For this review, take the finished solid that the model builds, in its own axes (mm). A direction names the side the tool comes from. Give positions to 0.01 mm unless a question says otherwise; leave off trailing zeros. Write each loop counter-clockwise with the first axis right and the second up, starting at its lowest first coordinate (ties: lowest second). Pieces come first, ordered by that corner, then holes. Notation, with made-up numbers: (17.25, -1) -> (61.25, -1) arc R21 cw to (61.25, 29) -> close; hole circle Ø7 at (33.25, -16). An arc over 180 degrees is marked (long way). Return JSON: item names as keys, results as strings.
from build123d import *

# Parameters (mm, degrees)
SKETCH_3_R          = 13
EXTRUDE_1_DEPTH     = 5
CUT_EXTRUDE_2_DEPTH = 2.5
SKETCH_11_R         = 10
EXTRUDE_2_DEPTH     = 15
SKETCH_6_R          = 2
CUT_EXTRUDE_3_DEPTH = 33
SKETCH_7_R          = 7
CUT_EXTRUDE_4_DEPTH = 23
CUT_EXTRUDE_6_DEPTH = 5
FILLET_1_R          = 1
SKETCH_10_W         = 2
SKETCH_10_H         = 14
CUT_EXTRUDE_7_DEPTH = 0.5


with BuildPart() as part:
    # ｽｹｯﾁ3 → ﾎﾞｽ - 押し出し1 (new body)
    with BuildSketch(Plane.XY):
        Circle(SKETCH_3_R)
    extrude(amount=EXTRUDE_1_DEPTH)

    # ｽｹｯﾁ2 → ｶｯﾄ - 押し出し2 (cut)
    with BuildSketch(Plane.XY):
        with BuildLine():
            Line((3.75, 6.495190528), (2.463350586, 13.926501921))
            ThreePointArc((2.463350586, 13.926501921), (0, 16), (-2.463350586, 13.926501921))
            Line((-2.463350586, 13.926501921), (-3.75, 6.495190528))
            Line((-3.75, 6.495190528), (-10.829029157, 9.096575147))
            ThreePointArc((-10.829029157, 9.096575147), (-13.856406461, 8), (-13.292379743, 4.829926775))
            Line((-13.292379743, 4.829926775), (-7.5, 0))
            Line((-7.5, 0), (-13.292379743, -4.829926775))
            ThreePointArc((-13.292379743, -4.829926775), (-13.856406461, -8), (-10.829029157, -9.096575147))
            Line((-10.829029157, -9.096575147), (-3.75, -6.495190528))
            Line((-3.75, -6.495190528), (-2.463350586, -13.926501921))
            ThreePointArc((-2.463350586, -13.926501921), (0, -16), (2.463350586, -13.926501921))
            Line((2.463350586, -13.926501921), (3.75, -6.495190528))
            Line((3.75, -6.495190528), (10.829029157, -9.096575147))
            ThreePointArc((10.829029157, -9.096575147), (13.856406461, -8), (13.292379743, -4.829926775))
            Line((13.292379743, -4.829926775), (7.5, 0))
            Line((7.5, 0), (13.292379743, 4.829926775))
            ThreePointArc((13.292379743, 4.829926775), (13.856406461, 8), (10.829029157, 9.096575147))
            Line((10.829029157, 9.096575147), (3.75, 6.495190528))
        make_face()
    extrude(amount=CUT_EXTRUDE_2_DEPTH, mode=Mode.SUBTRACT)

    # ｽｹｯﾁ11 → ﾎﾞｽ - 押し出し2 (add)
    with BuildSketch(Plane.XY.offset(5)):
        Circle(SKETCH_11_R)
    extrude(amount=EXTRUDE_2_DEPTH)

    # ｽｹｯﾁ5 → 回転1 (revolve)
    with BuildSketch(Plane(origin=(0, 0, 0), x_dir=(1, 0, 0), z_dir=(0, 1, 0))):
        Polygon((0, -20), (25, -20), (25, -22), (10, -22), (10, -30), (25, -30), (25, -32), (0, -32), align=None)
    revolve(axis=Axis((0, 0, 0), (0, 0, 1)))

    # ｽｹｯﾁ6 → ｶｯﾄ - 押し出し3 (cut, through all)
    with BuildSketch(Plane.XY.offset(32)):
        Circle(SKETCH_6_R)
    extrude(amount=-CUT_EXTRUDE_3_DEPTH, mode=Mode.SUBTRACT)

    # ｽｹｯﾁ7 → ｶｯﾄ - 押し出し4 (cut)
    with BuildSketch(Plane.XY.offset(32)):
        Circle(SKETCH_7_R)
    extrude(amount=-CUT_EXTRUDE_4_DEPTH, mode=Mode.SUBTRACT)

    # ｽｹｯﾁ9 → ｶｯﾄ - 押し出し6 (cut)
    with BuildSketch(Plane(origin=(0, 0, 30), x_dir=(-1, 0, 0), z_dir=(0, 0, -1))):
        Polygon((-3.843473937, -0.691164305), (-11.556925253, -9.883697623), (-7.726703038, -13.097635671), (-0.013251721, -3.905102354), align=None)
    cut_extrude_6 = extrude(amount=CUT_EXTRUDE_6_DEPTH, mode=Mode.SUBTRACT)

    # ﾐﾗｰ1: ｶｯﾄ - 押し出し6 across plane
    add(cut_extrude_6.mirror(Plane(origin=(0, 0, 0), x_dir=(0, 0, 1), z_dir=(1, 0, 0))), mode=Mode.SUBTRACT)

    # ﾌｨﾚｯﾄ1
    fillet_1_edges = [part.edges().sort_by_distance(p)[0] for p in [
        (4.308653161, -9.024162451, 27.5),
        (-4.308653161, -9.024162451, 27.5),
    ]]
    fillet(fillet_1_edges, radius=FILLET_1_R)

    # ｽｹｯﾁ10 → ｶｯﾄ - 押し出し7 (cut)
    with BuildSketch(Plane.XY.offset(32)):
        with Locations((0, 16)):
            Rectangle(SKETCH_10_W, SKETCH_10_H)
    extrude(amount=-CUT_EXTRUDE_7_DEPTH, mode=Mode.SUBTRACT)


solid = part.part
1. For faces 4 (the flat face through (1, 2, 9)), 5 (the flat face through (-6.67, 7.57, 1.23)), 6 (the flat face through (-9.96, 2.05, 1.23)), 7 (the flat face through (7.114, -4.589, 27.535)), 8 (the flat face through (6.76, 7.6, 1.23)), list the 3-axis set-ups (+Z, -Z, +X, -X, +Y, -Y) from which the entire face can be reached by the end or side of a thin tool; tool diameter is ignored.
Results found:
{"face 4": "+Z", "face 5": "-Z, -X", "face 6": "-Z", "face 7": "-Y", "face 8": "-Z, +X"}
2. Add section D-D, the plane x = -15. State the section outline as (y, z) points, plus the area to 3 significant figures.
Results found:
{"outline": "(-20, 20) -> (20, 20) -> (20, 22) -> (-20, 22) -> close; (-20, 30) -> (20, 30) -> (20, 32) -> (-20, 32) -> close", "area": "160 mm²"}
3. Add section B-B, the plane z = 28.5. State the section outline as (x, y) points, plus the area to 3 significant figures.
Results found:
{"outline": "(-8.14, -5.81) -> (-6.12, -3.4) arc R7 cw (long way) to (6.12, -3.4) -> (8.14, -5.81) arc R10 ccw (long way) to start; (-3.41, -7.96) arc R1 ccw to (-2.94, -9.56) arc R10 ccw to (2.94, -9.56) arc R1 ccw to (3.41, -7.96) -> (2.29, -6.62) arc R7 cw to (-2.29, -6.62) -> close", "area": "129 mm²"}
4. To check wall thickness, follow probe 1 along Z at (x, y) = (10, -4.5); probe 2 along Z at (x, y) = (-17.5, 10.5); probe 3 along Y at (x, z) = (0, 21). State the ranges of each line that lie inside material, in increasing order.
Results found:
{"probe 1": "z = 2.5 to 5, 20 to 22, 30 to 32", "probe 2": "z = 20 to 22, 30 to 32", "probe 3": "y = -25 to -7, 7 to 25"}
5. For pin 1 (12.5 mm diameter, centred on x = 0, y = 0, fed in from +Z); pin 2 (8 mm diameter, centred on y = 14.5, z = 23.5, fed in from -X); pin 3 (10 mm diameter, centred on y = -8, z = 21, fed in from -X); pin 4 (2.5 mm diameter, centred on x = 0, y = 0, fed in from +Z), all flat-tipped, find the tip position at first contact; note any pin that passes through.
Results found:
{"pin 1": "stops at z = 9", "pin 2": "stops at x = -22.55", "pin 3": "stops at x = -24.82", "pin 4": "passes through"}
6. Add section C-C, the plane y = 18. State the section outline as (x, z) points.
Results found:
{"outline": "(-17.35, 20) -> (17.35, 20) -> (17.35, 22) -> (-17.35, 22) -> close; (-17.35, 30) -> (17.35, 30) -> (17.35, 32) -> (1, 32) -> (1, 31.5) -> (-1, 31.5) -> (-1, 32) -> (-17.35, 32) -> close"}
7. The part is to be moulded in two halves that separate along Y. For faces 1 (the cylindrical face through (-2.17, -9.76, 12.4)), 2 (the flat face through (5.2, -5.2, 32)), 3 (the cylindrical face through (3.604, -8.898, 27.535)), say which applies: +Y half, -Y half, draft (parallel to the pull), parting line (faces both ways), or undercut.
Results found:
{"face 1": "parting line", "face 2": "draft", "face 3": "undercut"}
